CAD build for the part. Positions are in the model's coordinates, mm. A direction names the side the tool comes from. Round coordinates to 2 decimals unless told otherwise and drop trailing zeros. Order: outer loops, then holes, each group sorted by start corner. A loop starts at its lowest first (then second) coordinate and runs counter-clockwise, first axis right, second up. Notation, with made-up numbers: M 9.25,10.5 L 60.25,10.5 A20 ccw 60.25,40.5 Z; hole C -16,35.25 d5. An arc over 180 degrees is marked long. Answer as a JSON object with one key per item and string values.
```python
from build123d import *

# Parameters (mm, degrees)
EXTRUDE_1_DEPTH        = 294
FILLET_1_R             = 0.1
SKETCH_2_R             = 3.55
CUT_EXTRUDE_1_DEPTH    = 6
PATTERN_LINEAR_1_COUNT = 20
PATTERN_LINEAR_1_PITCH = 60
SKETCH_3_R             = 2.25
CUT_EXTRUDE_3_DEPTH    = 20
PATTERN_LINEAR_2_COUNT = 20
PATTERN_LINEAR_2_PITCH = 60


with BuildPart() as part:
    # Эскиз1 → Бобышка-Вытянуть1 (new body)
    with BuildSketch(Plane.XY):
        Polygon((-8.077815221, -6.752458719), (6.922184779, -6.752458719), (6.922184779, -1.152458719), (4.538392714, 1.231333345), (4.538392714, 2.234063435), (6.922184779, 4.617855499), (6.922184779, 5.117855499), (3.492498997, 8.547541281), (-4.64812944, 8.547541281), (-8.077815221, 5.117855499), (-8.077815221, 4.617855499), (-5.694023157, 2.234063435), (-5.694023157, 1.231333345), (-8.077815221, -1.152458719), align=None)
    extrude(amount=EXTRUDE_1_DEPTH)

    # Скругление1
    fillet_1_edges = [part.edges().sort_by_distance(p)[0] for p in [
        (6.922184779, -3.952458719, 294),
        (-6.885919189, 0.039437313, 0),
        (-5.694023157, 1.73269839, 0),
        (5.730288746, 0.039437313, 294),
        (-6.885919189, 3.425959467, 0),
        (-8.077815221, 4.867855499, 0),
        (-6.362972331, 6.83269839, 0),
        (-0.577815221, 8.547541281, 0),
        (5.207341888, 6.83269839, 0),
        (6.922184779, 4.867855499, 0),
        (5.730288746, 3.425959467, 0),
        (4.538392714, 1.73269839, 294),
        (4.538392714, 1.73269839, 0),
        (5.730288746, 0.039437313, 0),
        (6.922184779, -3.952458719, 0),
        (-0.577815221, -6.752458719, 0),
        (-8.077815221, -3.952458719, 0),
        (5.730288746, 3.425959467, 294),
        (6.922184779, 4.867855499, 294),
        (-8.077815221, -1.152458719, 147),
        (-5.694023157, 1.231333345, 147),
        (-5.694023157, 2.234063435, 147),
        (-8.077815221, 4.617855499, 147),
        (-8.077815221, 5.117855499, 147),
        (-4.64812944, 8.547541281, 147),
        (3.492498997, 8.547541281, 147),
        (6.922184779, 5.117855499, 147),
        (6.922184779, 4.617855499, 147),
        (4.538392714, 2.234063435, 147),
        (4.538392714, 1.231333345, 147),
        (6.922184779, -1.152458719, 147),
        (6.922184779, -6.752458719, 147),
        (-8.077815221, -6.752458719, 147),
        (5.207341888, 6.83269839, 294),
        (-0.577815221, 8.547541281, 294),
        (-6.362972331, 6.83269839, 294),
        (-8.077815221, 4.867855499, 294),
        (-6.885919189, 3.425959467, 294),
        (-8.077815221, -3.952458719, 294),
        (-5.694023157, 1.73269839, 294),
        (-6.885919189, 0.039437313, 294),
        (-0.577815221, -6.752458719, 294),
    ]]
    fillet(fillet_1_edges, radius=FILLET_1_R)

    # Эскиз2 → Вырез-Вытянуть1 (cut)
    with BuildSketch(Plane(origin=(0, 8.547541281, 0), x_dir=(1, 0, 0), z_dir=(0, 1, 0))):
        with Locations(Location((-0.647418762, -28.6, 0), (0, 0, 270))):
            Circle(SKETCH_2_R)
    cut_extrude_1 = extrude(amount=-CUT_EXTRUDE_1_DEPTH, mode=Mode.SUBTRACT)

    # Линейный массив1: Вырез-Вытянуть1 ×20
    with Locations(*[(0, 0, i * PATTERN_LINEAR_1_PITCH) for i in range(1, PATTERN_LINEAR_1_COUNT)]):
        add(cut_extrude_1, mode=Mode.SUBTRACT)

    # Эскиз3 → Вырез-Вытянуть3 (cut)
    with BuildSketch(Plane(origin=(0, 2.547541281, 0), x_dir=(1, 0, 0), z_dir=(0, 1, 0))):
        with Locations(Location((-0.647418762, -28.6, 0), (0, 0, 270))):
            Circle(SKETCH_3_R)
    cut_extrude_3 = extrude(amount=-CUT_EXTRUDE_3_DEPTH, mode=Mode.SUBTRACT)

    # Линейный массив2: Вырез-Вытянуть3 ×20
    with Locations(*[(0, 0, i * PATTERN_LINEAR_2_PITCH) for i in range(1, PATTERN_LINEAR_2_COUNT)]):
        add(cut_extrude_3, mode=Mode.SUBTRACT)


solid = part.part
```
Item 1: Wall check: line 1 along Z through (x, y) = (-0.75, -1.75); line 2 along Z through (x, y) = (0.25, 4); line 3 along Y through (x, z) = (-1, 31.5). Give the ranges that are in metal, low to high. Write a range as [from, to].
Worked answers:
{"line 1": "z = [0, 26.35], [30.85, 86.35], [90.85, 146.35], [150.85, 206.35], [210.85, 266.35], [270.85, 294]", "line 2": "z = [0, 25.17], [32.03, 85.17], [92.03, 145.17], [152.03, 205.17], [212.03, 265.17], [272.03, 294]", "line 3": "y = [-6.75, 2.55]"}
Item 2: Drop flat-ended pins along their axis: pin 1 Ø3.5 at (x, z) = (-0.65, 28.6) entering from -Y; pin 2 Ø1 at (y, z) = (2, 174) entering from -X; pin 3 Ø1.5 at (y, z) = (2.5, 98.5) entering from +X; pin 4 Ø6.5 at (x, z) = (-0.65, 208.6) entering from +Y. Give the stop position or say it passes through.
Worked answers:
{"pin 1": "passes through", "pin 2": "stops at x = -5.96", "pin 3": "stops at x = 5.55", "pin 4": "stops at y = 2.55"}
Item 3: 3-axis set-ups, long thin cutter, end or side, ignore diameter. For faces 1 (the cylindrical face through (-2.01, 5.59, 91.88)), 2 (the flat face through (-1, 1, 294)): which of +Z, -Z, +X, -X, +Y, -Y reach the whole face in a straight line?
Worked answers:
{"face 1": "+Y", "face 2": "+Z, +X, -X, +Y, -Y"}
Item 4: Saw through at A-A on y = -3.5. List the corners of the cut face in (x, z).
Worked answers:
{"outline": "M -8.08,0.1 A0.1 ccw -7.98,0 L 6.82,0 A0.1 ccw 6.92,0.1 L 6.92,293.9 A0.1 ccw 6.82,294 L -7.98,294 A0.1 ccw -8.08,293.9 Z; hole C -0.65,28.6 d4.5; hole C -0.65,88.6 d4.5; hole C -0.65,148.6 d4.5; hole C -0.65,208.6 d4.5; hole C -0.65,268.6 d4.5"}
Item 5: Two-plate mould, pull along X, no slides. Class faces 3 (the flat face through (6.922, -4, 145)), 4 (the flat face through (-0.5, 8.548, 144.9)), 5 (the cylindrical face through (-1.51, -2.04, 150.68)): released by +X, released by -X, zero draft, split by the parting line, or undercut.
Worked answers:
{"face 3": "released by +X", "face 4": "zero draft", "face 5": "undercut"}
Item 6: Saw through at B-B on z = 22. List the corners of the cut face in (x, y).
Worked answers:
{"outline": "M -8.08,-6.65 A0.1 ccw -7.98,-6.75 L 6.82,-6.75 A0.1 ccw 6.92,-6.65 L 6.92,-1.19 A0.1 ccw 6.89,-1.12 L 4.57,1.2 A0.1 cw 4.54,1.27 L 4.54,2.19 A0.1 cw 4.57,2.26 L 6.89,4.59 A0.1 ccw 6.92,4.66 L 6.92,5.08 A0.1 ccw 6.89,5.15 L 3.52,8.52 A0.1 ccw 3.45,8.55 L -4.61,8.55 A0.1 ccw -4.68,8.52 L -8.05,5.15 A0.1 ccw -8.08,5.08 L -8.08,4.66 A0.1 ccw -8.05,4.59 L -5.72,2.26 A0.1 cw -5.69,2.19 L -5.69,1.27 A0.1 cw -5.72,1.2 L -8.05,-1.12 A0.1 ccw -8.08,-1.19 Z"}
